```python
from build123d import *

# Parameters (mm, degrees)
F1_DEPTH = 3.95
F2_DEPTH = 3.45
F3_R     = 3.69999


# Not quite as in the source:
# - a fillet or chamfer is up to 0.001 mm smaller than in the source, because OpenCascade refuses the exact size


with BuildPart() as f1:
    # F0 (on Front) → F1 (new body, symmetric)
    with BuildSketch(Plane.XZ):
        with BuildLine():
            Line((21.3529593349, -11.1881163925), (-49.6470406651, -11.1881163925))
            Line((-49.6470406651, -11.1881163925), (-49.6470406651, -14.8881163925))
            Line((-49.6470406651, -14.8881163925), (-49.1470406651, -14.8881163925))
            ThreePointArc((-49.1470406651, -14.8881163925), (-46.1470406651, -11.8881163925), (-43.1470406651, -14.8881163925))
            Line((-43.1470406651, -14.8881163925), (-41.1470406651, -14.8881163925))
            ThreePointArc((-41.1470406651, -14.8881163925), (-38.1470406651, -11.8881163925), (-35.1470406651, -14.8881163925))
            Line((-35.1470406651, -14.8881163925), (-33.1470406651, -14.8881163925))
            ThreePointArc((-33.1470406651, -14.8881163925), (-30.1470406651, -11.8881163925), (-27.1470406651, -14.8881163925))
            Line((-27.1470406651, -14.8881163925), (-25.1470406651, -14.8881163925))
            ThreePointArc((-25.1470406651, -14.8881163925), (-22.1470406651, -11.8881163925), (-19.1470406651, -14.8881163925))
            Line((-19.1470406651, -14.8881163925), (-17.1470406651, -14.8881163925))
            ThreePointArc((-17.1470406651, -14.8881163925), (-14.1470406651, -11.8881163925), (-11.1470406651, -14.8881163925))
            Line((-11.1470406651, -14.8881163925), (-9.1470406651, -14.8881163925))
            ThreePointArc((-9.1470406651, -14.8881163925), (-6.1470406651, -11.8881163925), (-3.1470406651, -14.8881163925))
            Line((-3.1470406651, -14.8881163925), (-1.1470406651, -14.8881163925))
            ThreePointArc((-1.1470406651, -14.8881163925), (1.8529593349, -11.8881163925), (4.8529593349, -14.8881163925))
            Line((4.8529593349, -14.8881163925), (6.8529593349, -14.8881163925))
            ThreePointArc((6.8529593349, -14.8881163925), (9.8529593349, -11.8881163925), (12.8529593349, -14.8881163925))
            Line((12.8529593349, -14.8881163925), (14.8529593349, -14.8881163925))
            ThreePointArc((14.8529593349, -14.8881163925), (17.8529593349, -11.8881163925), (20.8529593349, -14.8881163925))
            Line((20.8529593349, -14.8881163925), (21.3529593349, -14.8881163925))
            Line((21.3529593349, -14.8881163925), (21.3529593349, -11.1881163925))
        make_face()
        with BuildLine():
            Line((-49.1470406651, -14.8881163925), (-49.6470406651, -14.8881163925))
            Line((-49.6470406651, -14.8881163925), (-49.6470406651, -18.5881163925))
            Line((-49.6470406651, -18.5881163925), (21.3529593349, -18.5881163925))
            Line((21.3529593349, -18.5881163925), (21.3529593349, -14.8881163925))
            Line((21.3529593349, -14.8881163925), (20.8529593349, -14.8881163925))
            ThreePointArc((20.8529593349, -14.8881163925), (17.8529593349, -17.8881163925), (14.8529593349, -14.8881163925))
            Line((14.8529593349, -14.8881163925), (12.8529593349, -14.8881163925))
            ThreePointArc((12.8529593349, -14.8881163925), (9.8529593349, -17.8881163925), (6.8529593349, -14.8881163925))
            Line((6.8529593349, -14.8881163925), (4.8529593349, -14.8881163925))
            ThreePointArc((4.8529593349, -14.8881163925), (1.8529593349, -17.8881163925), (-1.1470406651, -14.8881163925))
            Line((-1.1470406651, -14.8881163925), (-3.1470406651, -14.8881163925))
            ThreePointArc((-3.1470406651, -14.8881163925), (-6.1470406651, -17.8881163925), (-9.1470406651, -14.8881163925))
            Line((-9.1470406651, -14.8881163925), (-11.1470406651, -14.8881163925))
            ThreePointArc((-11.1470406651, -14.8881163925), (-14.1470406651, -17.8881163925), (-17.1470406651, -14.8881163925))
            Line((-17.1470406651, -14.8881163925), (-19.1470406651, -14.8881163925))
            ThreePointArc((-19.1470406651, -14.8881163925), (-22.1470406651, -17.8881163925), (-25.1470406651, -14.8881163925))
            Line((-25.1470406651, -14.8881163925), (-27.1470406651, -14.8881163925))
            ThreePointArc((-27.1470406651, -14.8881163925), (-30.1470406651, -17.8881163925), (-33.1470406651, -14.8881163925))
            Line((-33.1470406651, -14.8881163925), (-35.1470406651, -14.8881163925))
            ThreePointArc((-35.1470406651, -14.8881163925), (-38.1470406651, -17.8881163925), (-41.1470406651, -14.8881163925))
            Line((-41.1470406651, -14.8881163925), (-43.1470406651, -14.8881163925))
            ThreePointArc((-43.1470406651, -14.8881163925), (-46.1470406651, -17.8881163925), (-49.1470406651, -14.8881163925))
        make_face()
    extrude(amount=F1_DEPTH, both=True)

    # F0 (on Front) → F2 (join, symmetric)
    with BuildSketch(Plane.XZ):
        with BuildLine():
            ThreePointArc((-43.1470406651, -14.8881163925), (-46.1470406651, -11.8881163925), (-49.1470406651, -14.8881163925))
            Line((-49.1470406651, -14.8881163925), (-48.6470406651, -14.8881163925))
            ThreePointArc((-48.6470406651, -14.8881163925), (-46.1470406651, -12.3881163925), (-43.6470406651, -14.8881163925))
            Line((-43.6470406651, -14.8881163925), (-43.1470406651, -14.8881163925))
        make_face()
        with BuildLine():
            Line((-48.6470406651, -14.8881163925), (-49.1470406651, -14.8881163925))
            ThreePointArc((-49.1470406651, -14.8881163925), (-46.1470406651, -17.8881163925), (-43.1470406651, -14.8881163925))
            Line((-43.1470406651, -14.8881163925), (-43.6470406651, -14.8881163925))
            ThreePointArc((-43.6470406651, -14.8881163925), (-46.1470406651, -17.3881163925), (-48.6470406651, -14.8881163925))
        make_face()
        with BuildLine():
            ThreePointArc((14.8529593349, -14.8881163925), (17.8529593349, -17.8881163925), (20.8529593349, -14.8881163925))
            Line((20.8529593349, -14.8881163925), (20.3529593349, -14.8881163925))
            ThreePointArc((20.3529593349, -14.8881163925), (17.8529593349, -17.3881163925), (15.3529593349, -14.8881163925))
            Line((15.3529593349, -14.8881163925), (14.8529593349, -14.8881163925))
        make_face()
        with BuildLine():
            Line((20.3529593349, -14.8881163925), (20.8529593349, -14.8881163925))
            ThreePointArc((20.8529593349, -14.8881163925), (17.8529593349, -11.8881163925), (14.8529593349, -14.8881163925))
            Line((14.8529593349, -14.8881163925), (15.3529593349, -14.8881163925))
            ThreePointArc((15.3529593349, -14.8881163925), (17.8529593349, -12.3881163925), (20.3529593349, -14.8881163925))
        make_face()
        with BuildLine():
            ThreePointArc((-35.1470406651, -14.8881163925), (-38.1470406651, -11.8881163925), (-41.1470406651, -14.8881163925))
            Line((-41.1470406651, -14.8881163925), (-40.6470406651, -14.8881163925))
            ThreePointArc((-40.6470406651, -14.8881163925), (-38.1470406651, -12.3881163925), (-35.6470406651, -14.8881163925))
            Line((-35.6470406651, -14.8881163925), (-35.1470406651, -14.8881163925))
        make_face()
        with BuildLine():
            Line((-40.6470406651, -14.8881163925), (-41.1470406651, -14.8881163925))
            ThreePointArc((-41.1470406651, -14.8881163925), (-38.1470406651, -17.8881163925), (-35.1470406651, -14.8881163925))
            Line((-35.1470406651, -14.8881163925), (-35.6470406651, -14.8881163925))
            ThreePointArc((-35.6470406651, -14.8881163925), (-38.1470406651, -17.3881163925), (-40.6470406651, -14.8881163925))
        make_face()
        with BuildLine():
            ThreePointArc((6.8529593349, -14.8881163925), (9.8529593349, -17.8881163925), (12.8529593349, -14.8881163925))
            Line((12.8529593349, -14.8881163925), (12.3529593349, -14.8881163925))
            ThreePointArc((12.3529593349, -14.8881163925), (9.8529593349, -17.3881163925), (7.3529593349, -14.8881163925))
            Line((7.3529593349, -14.8881163925), (6.8529593349, -14.8881163925))
        make_face()
        with BuildLine():
            Line((12.3529593349, -14.8881163925), (12.8529593349, -14.8881163925))
            ThreePointArc((12.8529593349, -14.8881163925), (9.8529593349, -11.8881163925), (6.8529593349, -14.8881163925))
            Line((6.8529593349, -14.8881163925), (7.3529593349, -14.8881163925))
            ThreePointArc((7.3529593349, -14.8881163925), (9.8529593349, -12.3881163925), (12.3529593349, -14.8881163925))
        make_face()
        with BuildLine():
            ThreePointArc((-27.1470406651, -14.8881163925), (-30.1470406651, -11.8881163925), (-33.1470406651, -14.8881163925))
            Line((-33.1470406651, -14.8881163925), (-32.6470406651, -14.8881163925))
            ThreePointArc((-32.6470406651, -14.8881163925), (-30.1470406651, -12.3881163925), (-27.6470406651, -14.8881163925))
            Line((-27.6470406651, -14.8881163925), (-27.1470406651, -14.8881163925))
        make_face()
        with BuildLine():
            Line((-32.6470406651, -14.8881163925), (-33.1470406651, -14.8881163925))
            ThreePointArc((-33.1470406651, -14.8881163925), (-30.1470406651, -17.8881163925), (-27.1470406651, -14.8881163925))
            Line((-27.1470406651, -14.8881163925), (-27.6470406651, -14.8881163925))
            ThreePointArc((-27.6470406651, -14.8881163925), (-30.1470406651, -17.3881163925), (-32.6470406651, -14.8881163925))
        make_face()
        with BuildLine():
            ThreePointArc((-1.1470406651, -14.8881163925), (1.8529593349, -17.8881163925), (4.8529593349, -14.8881163925))
            Line((4.8529593349, -14.8881163925), (4.3529593349, -14.8881163925))
            ThreePointArc((4.3529593349, -14.8881163925), (1.8529593349, -17.3881163925), (-0.6470406651, -14.8881163925))
            Line((-0.6470406651, -14.8881163925), (-1.1470406651, -14.8881163925))
        make_face()
        with BuildLine():
            Line((4.3529593349, -14.8881163925), (4.8529593349, -14.8881163925))
            ThreePointArc((4.8529593349, -14.8881163925), (1.8529593349, -11.8881163925), (-1.1470406651, -14.8881163925))
            Line((-1.1470406651, -14.8881163925), (-0.6470406651, -14.8881163925))
            ThreePointArc((-0.6470406651, -14.8881163925), (1.8529593349, -12.3881163925), (4.3529593349, -14.8881163925))
        make_face()
        with BuildLine():
            ThreePointArc((-19.1470406651, -14.8881163925), (-22.1470406651, -11.8881163925), (-25.1470406651, -14.8881163925))
            Line((-25.1470406651, -14.8881163925), (-24.6470406651, -14.8881163925))
            ThreePointArc((-24.6470406651, -14.8881163925), (-22.1470406651, -12.3881163925), (-19.6470406651, -14.8881163925))
            Line((-19.6470406651, -14.8881163925), (-19.1470406651, -14.8881163925))
        make_face()
        with BuildLine():
            Line((-24.6470406651, -14.8881163925), (-25.1470406651, -14.8881163925))
            ThreePointArc((-25.1470406651, -14.8881163925), (-22.1470406651, -17.8881163925), (-19.1470406651, -14.8881163925))
            Line((-19.1470406651, -14.8881163925), (-19.6470406651, -14.8881163925))
            ThreePointArc((-19.6470406651, -14.8881163925), (-22.1470406651, -17.3881163925), (-24.6470406651, -14.8881163925))
        make_face()
        with BuildLine():
            ThreePointArc((-9.1470406651, -14.8881163925), (-6.1470406651, -17.8881163925), (-3.1470406651, -14.8881163925))
            Line((-3.1470406651, -14.8881163925), (-3.6470406651, -14.8881163925))
            ThreePointArc((-3.6470406651, -14.8881163925), (-6.1470406651, -17.3881163925), (-8.6470406651, -14.8881163925))
            Line((-8.6470406651, -14.8881163925), (-9.1470406651, -14.8881163925))
        make_face()
        with BuildLine():
            Line((-3.6470406651, -14.8881163925), (-3.1470406651, -14.8881163925))
            ThreePointArc((-3.1470406651, -14.8881163925), (-6.1470406651, -11.8881163925), (-9.1470406651, -14.8881163925))
            Line((-9.1470406651, -14.8881163925), (-8.6470406651, -14.8881163925))
            ThreePointArc((-8.6470406651, -14.8881163925), (-6.1470406651, -12.3881163925), (-3.6470406651, -14.8881163925))
        make_face()
        with BuildLine():
            ThreePointArc((-11.1470406651, -14.8881163925), (-14.1470406651, -11.8881163925), (-17.1470406651, -14.8881163925))
            Line((-17.1470406651, -14.8881163925), (-16.6470406651, -14.8881163925))
            ThreePointArc((-16.6470406651, -14.8881163925), (-14.1470406651, -12.3881163925), (-11.6470406651, -14.8881163925))
            Line((-11.6470406651, -14.8881163925), (-11.1470406651, -14.8881163925))
        make_face()
        with BuildLine():
            Line((-16.6470406651, -14.8881163925), (-17.1470406651, -14.8881163925))
            ThreePointArc((-17.1470406651, -14.8881163925), (-14.1470406651, -17.8881163925), (-11.1470406651, -14.8881163925))
            Line((-11.1470406651, -14.8881163925), (-11.6470406651, -14.8881163925))
            ThreePointArc((-11.6470406651, -14.8881163925), (-14.1470406651, -17.3881163925), (-16.6470406651, -14.8881163925))
        make_face()
    extrude(amount=F2_DEPTH, both=True)

    # F3 (radius 3.7 in the source; OpenCascade refuses exactly that, so slightly less here)
    f3_edges = [f1.edges().sort_by_distance(p)[0] for p in [
        (21.352959, 0, -11.188116),
        (21.352959, 0, -18.588116),
        (-49.647041, 0, -11.188116),
        (-49.647041, 0, -18.588116),
    ]]
    fillet(f3_edges, radius=F3_R)


solid = f1.part
```
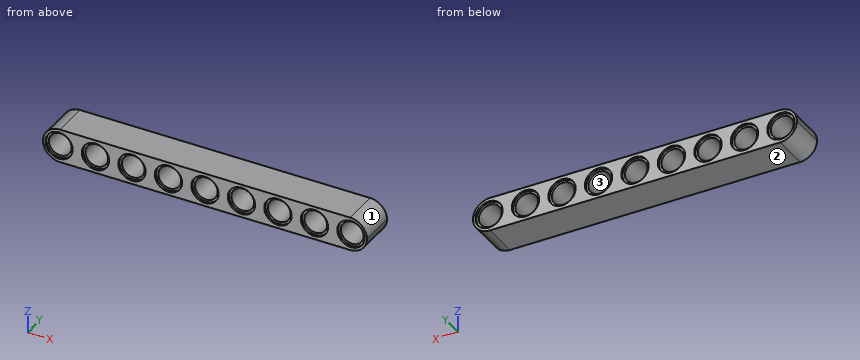
For this review, take the finished solid that the model builds, in its own axes (mm). Face numbers are marked on the shaded views. Give positions to 0.01 mm unless a question says otherwise; leave off trailing zeros. Write each loop counter-clockwise with the first axis right and the second up, starting at its lowest first coordinate (ties: lowest second). Pieces come first, ordered by that corner, then holes.
Item 1: Take a section at C-C (x = -29.5). Give the boundary of the cut face in (y, z).
Item 2: Wall thickness on probe 1 along Z at (x, y) = (10, 0); probe 2 along Y at (x, z) = (-30, -17.75); probe 3 along X at (y, z) = (-3, -18): over which ranges is each line inside the solid? List them lowest first.
Item 3: Take a section at B-B (x = 10). Give the boundary of the cut face in (y, z), and give its area (3 significant figures).
Item 4: Take a section at A-A (y = -0.75). Give the number of separate pieces and of enclosed holes in the cut face, and give its area (3 significant figures).
Item 5: Insertion check: P1, Ø3, axis at x = 9.5, z = -15, coming from the -Y side; P2, Ø1, axis at y = -1, z = -16.5, coming from the +X side. Each pin has a flat end and moves straight along its axis. Give the tip position at first contact, or say it passes through.
Item 6: The part is to be moulded in two halves that separate along Z. For the marked faces 1, 2 and 3, say which applies: +Z half, -Z half, draft (parallel to the pull), parting line (faces both ways), or undercut.
Established:
1. outline: (-3.95, -18.59) - (3.95, -18.59) - (3.95, -17.82) - (3.45, -17.82) - (3.45, -17.3) - (-3.45, -17.3) - (-3.45, -17.82) - (-3.95, -17.82) - close; (-3.95, -11.96) - (-3.45, -11.96) - (-3.45, -12.47) - (3.45, -12.47) - (3.45, -11.96) - (3.95, -11.96) - (3.95, -11.19) - (-3.95, -11.19) - close
2. probe 1: z = -18.59 to -17.38, -12.39 to -11.19
2. probe 2: y = -3.45 to 3.45
2. probe 3: x = -47.95 to 19.65
3. outline: (-3.95, -18.59) - (3.95, -18.59) - (3.95, -17.88) - (3.45, -17.88) - (3.45, -17.38) - (-3.45, -17.38) - (-3.45, -17.88) - (-3.95, -17.88) - close; (-3.95, -11.89) - (-3.45, -11.89) - (-3.45, -12.39) - (3.45, -12.39) - (3.45, -11.89) - (3.95, -11.89) - (3.95, -11.19) - (-3.95, -11.19) - close
3. area: 18.0 mm2
4. separate pieces: 1
4. enclosed holes: 9
4. area: 337 mm2
5. P1: passes through
5. P2: stops at x = 21.18
6. face 1: +Z half
6. face 2: -Z half
6. face 3: undercut
